```python
from build123d import *

# Parameters (mm, degrees)
F1_DEPTH = 127.6796478778
F2_R     = 10.0565925357
F3_DEPTH = 204.0422167629
F4_R     = 36.1265659612
F5_DEPTH = 25.4


with BuildPart() as f1:
    # F0 (on Front) → F1 (new body)
    with BuildSketch(Plane.XZ):
        Polygon((28.2338894904, 185.2392554283), (-54.3228834867, 89.0406146646), (-54.3228834867, 68.8263475895), (75.0374570489, 100.4021242261), align=None)
    extrude(amount=F1_DEPTH)

    # F2 (on face) → F3 (join)
    with BuildSketch(Plane(origin=(0, 0, 0), x_dir=(-1, 0, 0), z_dir=(0, 1, 0))):
        with Locations((0, 106.0985550284)):
            Circle(F2_R)
    extrude(amount=F3_DEPTH)

    # F4 (on face) → F5 (cut)
    with BuildSketch(Plane(origin=(99.9939788149, 0, 55.1654078419), x_dir=(0, 1, 0), z_dir=(0.8755913279, 0, 0.4830526126))):
        with Locations((-74.4225531816, 51.6641896083)):
            Circle(F4_R)
    extrude(amount=-F5_DEPTH, mode=Mode.SUBTRACT)


solid = f1.part
```
Design review of the part built by this model. Coordinates are the model's own, in mm. A direction names the side the tool comes from. Round coordinates to 2 decimals unless told otherwise and drop trailing zeros. Write each loop counter-clockwise with the first axis right and the second up, starting at its lowest first coordinate (ties: lowest second). Pieces come first, ordered by that corner, then holes.
Item 1: We need section D-D on y = 98.5. Write out the cut boundary in (x, z), and give its area (3 significant figures).
Item 2: We need section A-A on y = -33.5. Write out the cut boundary in (x, z).
Item 3: The part is to be moulded in two halves that separate along Y. For faces 3 (the flat face through (9, -127.68, 115)), 4 (the cylindrical face through (46.63, -73.63, 125.98)), 5 (the flat face through (43.88, -74.92, 104.3)), 6 (the flat face through (-12.47, -62.95, 137.81)), say which applies: +Y half, -Y half, draft (parallel to the pull), parting line (faces both ways), or undercut.
Item 4: We need section C-C on x = 18.5. Write out the cut boundary in (y, z), and give its area (3 significant figures).
Item 5: For faces 1 (the flat face through (-54.323, -63, 79)), 2 (the cylindrical face through (2.18, 100.59, 96.28)), list the 3-axis set-ups (+Z, -Z, +X, -X, +Y, -Y) from which the entire face can be reached by the end or side of a thin tool; tool diameter is ignored.
Item 6: For probe 1 along Y at (x, z) = (-13, 98.5); probe 2 along Z at (x, y) = (45.5, -91.5); probe 3 along X at (y, z) = (103, 107), list the stretches that pass through material, from the lowest coordinate up.
Item 7: We need section B-B on x = 0. Write out the cut boundary in (y, z).
Item 8: Clearance check with flat-ended pins moving along their axes: pin 1 Ø3 at (x, z) = (48.5, 101) entering from +Y; pin 2 Ø12 at (x, y) = (-39.5, -64) entering from +Z; pin 3 Ø3 at (x, y) = (53, 1) entering from +Z. State where each tip first meets the part, or that it passes through.
Returned:
1. outline: circle Ø20.11 at (0, 106.1)
1. area: 318 mm2
2. outline: (-54.32, 68.83) - (75.04, 100.4) - (28.23, 185.24) - (-54.32, 89.04) - close
3. face 3: -Y half
3. face 4: undercut
3. face 5: undercut
3. face 6: draft
4. outline: (-127.68, 86.6) - (0, 86.6) - (0, 173.9) - (-127.68, 173.9) - close
4. area: 11,100 mm2
5. face 1: +Z, -Z, -X, +Y, -Y
5. face 2: +Y
6. probe 1: y = -127.68 to 0
6. probe 2: z = 93.19 to 101.36, 120.47 to 153.94
6. probe 3: x = -10.02 to 10.02
7. outline: (-127.68, 82.09) - (0, 82.09) - (0, 96.04) - (204.04, 96.04) - (204.04, 116.16) - (0, 116.16) - (0, 152.34) - (-127.68, 152.34) - close
8. pin 1: stops at y = 0
8. pin 2: stops at z = 113.3
8. pin 3: stops at z = 142.37
